Could you check a few things on this model? Use its own coordinates, in mm. A direction names the side the tool comes from. Round coordinates to 2 decimals unless told otherwise and drop trailing zeros. Loops run counter-clockwise (first coordinate to the right, second up) from the corner with the lowest first, then second, coordinate; pieces in that order, holes last.
from build123d import *

# Parameters (mm, degrees)
SKETCH_1_W          = 18
SKETCH_1_H          = 18
EXTRUDE_1_DEPTH     = 6
SKETCH_3_W          = 20
SKETCH_3_H          = 20
EXTRUDE_2_DEPTH     = 2
FILLET_1_R          = 1
CUT_EXTRUDE_2_DEPTH = 1


with BuildPart() as part:
    # 草图1 → 凸台-拉伸1 (new body)
    with BuildSketch(Plane.XY):
        Rectangle(SKETCH_1_W, SKETCH_1_H)
    extrude(amount=EXTRUDE_1_DEPTH)

    # 草图3 → 凸台-拉伸2 (add)
    with BuildSketch(Plane.XY.offset(6)):
        Rectangle(SKETCH_3_W, SKETCH_3_H)
    extrude(amount=EXTRUDE_2_DEPTH)

    # 圆角1
    fillet_1_edges = [part.edges().sort_by_distance(p)[0] for p in [
        (10, -10, 7),
        (10, 10, 7),
        (-10, 10, 7),
        (-10, -10, 7),
    ]]
    fillet(fillet_1_edges, radius=FILLET_1_R)

    # 草图5 → 切除-拉伸2 (cut)
    with BuildSketch(Plane.XY.offset(8)):
        with BuildLine():
            Line((-7.204561004, 1.879394949), (-8.234522443, -1.859506165))
            Line((-8.234522443, -1.859506165), (-5.723109619, -1.859506165))
            ThreePointArc((-5.723109619, -1.859506165), (-5.218538697, -1.632457047), (-4.78861912, -1.284157931))
            Line((-4.78861912, -1.284157931), (-4.947111275, -1.859506165))
            Line((-4.947111275, -1.859506165), (-3.352787404, -1.859506165))
            ThreePointArc((-3.352787404, -1.859506165), (-2.759972983, -1.585355224), (-2.30360072, -1.118116491))
            Line((-2.30360072, -1.118116491), (-1.497804292, 1.879394949))
            Line((-1.497804292, 1.879394949), (-2.436323584, 1.879394949))
            Line((-2.436323584, 1.879394949), (-3.079504637, -0.513197642))
            ThreePointArc((-3.079504637, -0.513197642), (-3.32542599, -0.827982147), (-3.696433402, -0.976036515))
            Line((-3.696433402, -0.976036515), (-4.666789972, -0.976036515))
            Line((-4.666789972, -0.976036515), (-3.880199418, 1.879394949))
            Line((-3.880199418, 1.879394949), (-4.81871871, 1.879394949))
            Line((-4.81871871, 1.879394949), (-5.477810253, -0.513197642))
            ThreePointArc((-5.477810253, -0.513197642), (-5.7047457, -0.820725721), (-6.053961641, -0.976036515))
            Line((-6.053961641, -0.976036515), (-7.003517302, -0.976036515))
            Line((-7.003517302, -0.976036515), (-6.216926747, 1.879394949))
            Line((-6.216926747, 1.879394949), (-7.204561004, 1.879394949))
        make_face()
        with BuildLine():
            Line((-0.857127264, 1.088853082), (-0.644612375, 1.879394949))
            Line((-0.644612375, 1.879394949), (2.196209614, 1.879394949))
            ThreePointArc((2.196209614, 1.879394949), (2.612575491, 1.570775142), (2.803252851, 1.088853082))
            Line((2.803252851, 1.088853082), (1.498562909, 1.088853082))
            Line((1.498562909, 1.088853082), (1.498562909, 0.920146657))
            Line((1.498562909, 0.920146657), (0.751331627, -1.859506165))
            Line((0.751331627, -1.859506165), (-0.236975463, -1.859506165))
            Line((-0.236975463, -1.859506165), (0.463990432, 0.748042361))
            ThreePointArc((0.463990432, 0.748042361), (0.35056842, 0.970657535), (0.130450539, 1.088853082))
            Line((0.130450539, 1.088853082), (-0.857127264, 1.088853082))
        make_face()
        with BuildLine():
            Line((3.92496477, 1.879394949), (2.919866632, -1.859506165))
            Line((2.919866632, -1.859506165), (3.879786702, -1.859506165))
            Line((3.879786702, -1.859506165), (4.67236995, 1.088853082))
            Line((4.67236995, 1.088853082), (6.439189541, 1.088853082))
            ThreePointArc((6.439189541, 1.088853082), (6.74191311, 0.79302609), (6.831437365, 0.379334689))
            Line((6.831437365, 0.379334689), (4.973337874, 0.379334689))
            Line((4.973337874, 0.379334689), (4.777076341, -0.350745725))
            Line((4.777076341, -0.350745725), (6.123295998, -0.350745725))
            ThreePointArc((6.123295998, -0.350745725), (6.221884558, -0.372626448), (6.288711068, -0.448340962))
            Line((6.288711068, -0.448340962), (6.481965147, -0.894824524))
            ThreePointArc((6.481965147, -0.894824524), (6.543334906, -1.375731382), (6.574951556, -1.859506165))
            Line((6.574951556, -1.859506165), (7.717356009, -1.859506165))
            ThreePointArc((7.717356009, -1.859506165), (7.71253802, -0.938991532), (7.378394237, -0.081251283))
            Line((7.378394237, -0.081251283), (8.199786702, -0.081251283))
            ThreePointArc((8.199786702, -0.081251283), (7.934816182, 1.144935193), (6.917805112, 1.879394949))
            Line((6.917805112, 1.879394949), (3.92496477, 1.879394949))
        make_face()
    extrude(amount=-CUT_EXTRUDE_2_DEPTH, mode=Mode.SUBTRACT)


solid = part.part
Item 1: Will these pins go through, and if not, where does the flat tip stop? pin 1 (6 mm diameter, centred on x = 4.5, y = 7, fed in from -Z); pin 2 (1.8 mm diameter, centred on y = 1.5, z = 2, fed in from -X); pin 3 (2 mm diameter, centred on x = 6, z = 3, fed in from +Y).
Results list:
pin 1: stops at z = 0
pin 2: stops at x = -9
pin 3: stops at y = 9
Item 2: We'd pull the mould along X, two halves only. Please class faces 1 (the cylindrical face through (-9.715, -9.699, 7.014)), 2 (the flat face through (-5.144, 0.7, 7.507)), 3 (the flat face through (0, 9, 3)): released by +X, released by -X, zero draft, split by the parting line, or undercut.
Results list:
face 1: released by -X
face 2: undercut
face 3: zero draft
Item 3: If we section it at A-A, the plane y = 3: Please give me the cut outline in (x, z).
Results list:
outline: (-10, 6) - (-9, 6) - (-9, 0) - (9, 0) - (9, 6) - (10, 6) - (10, 8) - (-10, 8) - close
Item 4: If we section it at C-C, the plane z = 2: Please give me the cut outline in (x, y), then the cut area to 3 significant figures.
Results list:
outline: (-9, -9) - (9, -9) - (9, 9) - (-9, 9) - close
area: 324 mm2
Item 5: If I drill on line 1 along X through (y, z) = (7.25, 5); line 2 along Y through (x, z) = (7.5, 7.25), over which ranges is the centre line in solid material (lowest first)?
Results list:
line 1: x = -9 to 9
line 2: y = -10 to -1.86, -0.3 to -0.08, 1.6 to 10
Item 6: For faces 4 (the flat face through (-9, 0, 3)), 5 (the flat face through (0, -9, 3)), 6 (the flat face through (0, 0, 8)), 7 (the cylindrical face through (7.945, 1.13, 7.507)), which set-ups out of +Z, -Z, +X, -X, +Y, -Y let a thin tool reach every point of the face, with its end or its side?
Results list:
face 4: -Z, -X, +Y, -Y
face 5: -Z, +X, -X, -Y
face 6: +Z, +X, -X, +Y, -Y
face 7: +Z
Item 7: If we section it at D-D, the plane x = 3.25: Please give me the cut outline in (y, z).
Results list:
outline: (-10, 6) - (-9, 6) - (-9, 0) - (9, 0) - (9, 6) - (10, 6) - (10, 8) - (-0.63, 8) - (-0.63, 7) - (-1.86, 7) - (-1.86, 8) - (-10, 8) - close
Item 8: If we section it at B-B, the plane x = -2: Please give me the cut outline in (y, z), then the cut area to 3 significant figures.
Results list:
outline: (-10, 6) - (-9, 6) - (-9, 0) - (9, 0) - (9, 6) - (10, 6) - (10, 8) - (1.88, 8) - (1.88, 7) - (0.01, 7) - (0.01, 8) - (-10, 8) - close
area: 146 mm2
